```python
from build123d import *

# Parameters (mm, degrees)
F0_R     = 11
F0_R_2   = 4
F1_DEPTH = 4
F2_R     = 9
F2_R_2   = 6
F3_DEPTH = 0.8
F4_SIZE  = 0.5


# Not quite as in the source:
# - a pattern or mirror of a feature is missing from the dataset's text; its kind, count and spacing are read off the source's solid


with BuildPart() as f1:
    # F0 (on Top) → F1 (new body, symmetric)
    with BuildSketch(Plane.XY):
        Circle(F0_R)
        Circle(F0_R_2, mode=Mode.SUBTRACT)
    extrude(amount=F1_DEPTH, both=True)

    # F2 (on face) → F3 (cut)
    with BuildSketch(Plane.XY.offset(4)):
        Circle(F2_R)
        Circle(F2_R_2, mode=Mode.SUBTRACT)
    f3 = extrude(amount=-F3_DEPTH, mode=Mode.SUBTRACT)

    # F3_copies: F3 across plane
    add(f3.mirror(Plane(origin=(0, 0, 0), x_dir=(-1, 0, 0), z_dir=(0, 0, -1))), mode=Mode.SUBTRACT)

    # F4
    f4_edges = [f1.edges().sort_by_distance(p)[0] for p in [
        (-11, 0, 4),
        (-11, 0, -4),
    ]]
    chamfer(f4_edges, length=F4_SIZE)


solid = f1.part
```
The listing builds one solid part. Answer for the finished solid, in the listing's coordinates (mm). A direction names the side the tool comes from. Coordinates: 2 decimals unless noted, no trailing zeros. Order: outer loops, then holes, each group sorted by start corner. A loop starts at its lowest first (then second) coordinate and runs counter-clockwise, first axis right, second up. Notation, with made-up numbers: M -15,70.5 L 35,70.5 A26 ccw 35,108.5 Z; hole C 24.25,19.25 d4. An arc over 180 degrees is marked long. Answer as a JSON object with one key per item and string values. Group by question number.
1. Section A-A on y = 0 is taken. Write down the section's boundary in (x, z), then the cut area to 3 significant figures.
2. Section C-C on z = -2.5 is taken. Write down the section's boundary in (x, y).
3. Determine the mould class of faces 4 (the flat face through (2, -6, 3.2)), 5 (the flat face through (-1.42, -3.92, 4)), 6 (the cylindrical face through (-2.38, -10.74, 0.05)) for opening direction X: released by +X, released by -X, zero draft, split by the parting line, or undercut.
4. A tool of negligible diameter and unlimited length cuts with its end or side. For faces 1 (the cylindrical face through (-5.994, 0.264, 3.606)), 2 (the flat face through (-1.42, -3.92, -4)), 3 (the cylindrical face through (-1.172, 8.923, -3.606)), from which of +Z, -Z, +X, -X, +Y, -Y can it reach the whole face along a straight path? Write none if from no direction.
5. Flat-ended cylindrical pins translate along their axes: P1, Ø2, axis at y = -2, z = 2, coming from the +X side; P2, Ø1.5, axis at y = -4, z = -2.5, coming from the -X side; P3, Ø9, axis at x = -1, y = 0.5, coming from the +Z side; P4, Ø1.5, axis at y = -8.5, z = 1.5, coming from the -X side. Find the tip coordinate at first contact, or state that the pin passes through.
6. Straight lines are drawn through the part: line 1 (Y direction, x = 0, z = -3.4); line 2 (Y direction, x = 0, z = 3.8); line 3 (Y direction, x = 0, z = 1). For each, find the intervals that lie inside material, in ascending order.
Values follow:
{
 "1": {"outline": "M -11,-3.5 L -10.5,-4 L -9,-4 L -9,-3.2 L -6,-3.2 L -6,-4 L -4,-4 L -4,4 L -6,4 L -6,3.2 L -9,3.2 L -9,4 L -10.5,4 L -11,3.5 Z; M 4,-4 L 6,-4 L 6,-3.2 L 9,-3.2 L 9,-4 L 10.5,-4 L 11,-3.5 L 11,3.5 L 10.5,4 L 9,4 L 9,3.2 L 6,3.2 L 6,4 L 4,4 Z", "area": "102 mm2"},
 "2": {"outline": "C 0,0 d22; hole C 0,0 d8"},
 "3": {"face 4": "undercut", "face 5": "zero draft", "face 6": "split by the parting line"},
 "4": {"face 1": "+Z", "face 2": "-Z, +X, -X, +Y, -Y", "face 3": "-Z"},
 "5": {"P1": "x = 10.95", "P2": "x = -10.51", "P3": "z = 4", "P4": "x = -7.81"},
 "6": {"line 1": "-11 to -9, -6 to -4, 4 to 6, 9 to 11", "line 2": "-10.7 to -9, -6 to -4, 4 to 6, 9 to 10.7", "line 3": "-11 to -4, 4 to 11"}
}
